CAD build for the part. Positions are in the model's coordinates, mm. Face numbers are marked on the shaded views. A direction names the side the tool comes from. Round coordinates to 2 decimals unless told otherwise and drop trailing zeros. Order: outer loops, then holes, each group sorted by start corner. A loop starts at its lowest first (then second) coordinate and runs counter-clockwise, first axis right, second up. Notation, with made-up numbers: M 23,10.25 L 62,10.25 A16 ccw 62,39.25 Z; hole C -16,5 d9. An arc over 180 degrees is marked long. Put each result on its own line as item: value.
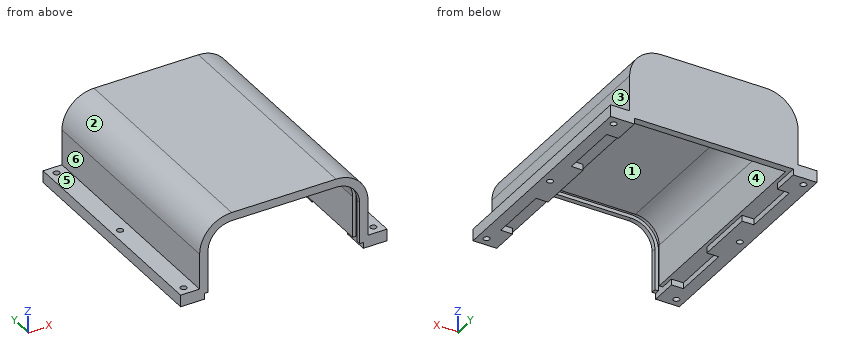
```python
from build123d import *

# Parameters (mm, degrees)
SKETCH_W        = 174
SKETCH_H        = 195
SKETCH_R        = 2.6
PAD_DEPTH       = 10
PAD001_DEPTH    = 195
POCKET_DEPTH    = 5
POCKET_FACE10_W = 195
POCKET_FACE10_H = 128
POCKET001_DEPTH = 5
PAD003_DEPTH    = 6
POCKET003_DEPTH = 10
PAD006_DEPTH    = 4


with BuildPart() as part:
    # Sketch → Pad (new body)
    with BuildSketch(Plane.XY):
        Rectangle(SKETCH_W, SKETCH_H)
        with Locations((80, 90)):
            Circle(SKETCH_R, mode=Mode.SUBTRACT)
        with Locations((-80, 90)):
            Circle(SKETCH_R, mode=Mode.SUBTRACT)
        with Locations((-80, -90)):
            Circle(SKETCH_R, mode=Mode.SUBTRACT)
        with Locations((80, -90)):
            Circle(SKETCH_R, mode=Mode.SUBTRACT)
        with Locations((-80, 0)):
            Circle(SKETCH_R, mode=Mode.SUBTRACT)
        with Locations((80, 0)):
            Circle(SKETCH_R, mode=Mode.SUBTRACT)
    extrude(amount=PAD_DEPTH)

    # Sketch001 (on Face3 of Pad) → Pad001 (join)
    with BuildSketch(Plane.XZ.offset(97.5)):
        with BuildLine():
            Line((-64, 10), (-64, 40))
            ThreePointArc((-44, 60), (-58.142136, 54.142136), (-64, 40))
            Line((-44, 60), (44, 60))
            ThreePointArc((64, 40), (58.142136, 54.142136), (44, 60))
            Line((64, 40), (64, 10))
            Line((64, 10), (71, 10))
            Line((71, 40), (71, 10))
            ThreePointArc((71, 40), (63.091883, 59.091883), (44, 67))
            Line((-44, 67), (44, 67))
            ThreePointArc((-44, 67), (-63.091883, 59.091883), (-71, 40))
            Line((-71, 10), (-71, 40))
            Line((-64, 10), (-71, 10))
        make_face()
    extrude(amount=-PAD001_DEPTH)

    # Sketch003 (on Face4 of Pad001) → Pocket (cut)
    with BuildSketch(Plane(origin=(0, 0, 0), x_dir=(1, 0, 0), z_dir=(0, 0, -1))):
        Polygon((-67, 97.5), (67, 97.5), (67, 75), (77, 75), (77, 25), (67, 25), (67, 0), (67, -25), (77, -25), (77, -75), (67, -75), (67, -97.5), (-67, -97.5), (-67, -75), (-77, -75), (-77, -25), (-67, -25), (-67, 0), (-67, 25), (-77, 25), (-77, 75), (-67, 75), align=None)
    extrude(amount=-POCKET_DEPTH, mode=Mode.SUBTRACT)

    # Pocket Face10 → Pocket001 (cut)
    with BuildSketch(Plane(origin=(0, 0, 10), x_dir=(0, 1, 0), z_dir=(0, 0, 1))):
        Rectangle(POCKET_FACE10_W, POCKET_FACE10_H)
    extrude(amount=-POCKET001_DEPTH, mode=Mode.SUBTRACT)

    # Sketch005 (on Face6 of Pocket001) → Pad003 (join)
    with BuildSketch(Plane(origin=(0, 97.5, 0), x_dir=(-1, 0, 0), z_dir=(0, 1, 0))):
        with BuildLine():
            Line((-64, 5), (64, 5))
            Line((64, 40), (64, 5))
            ThreePointArc((64, 40), (58.142143, 54.142129), (44.00002, 60))
            Line((-44, 60), (44.00002, 60))
            ThreePointArc((-44, 60), (-58.142136, 54.142136), (-64, 40))
            Line((-64, 40), (-64, 5))
        make_face()
    extrude(amount=-PAD003_DEPTH)

    # Sketch006 (on Face30 of Pad003) → Pocket003 (cut)
    with BuildSketch(Plane.XZ.offset(97.5)):
        with BuildLine():
            ThreePointArc((-44, 63), (-60.263456, 56.263456), (-67, 40))
            Line((-67, 40), (-67, 0))
            Line((-67, 0), (67, 0))
            Line((67, 0), (67, 40))
            ThreePointArc((67, 40), (60.263456, 56.263456), (44, 63))
            Line((-44, 63), (44, 63))
        make_face()
    extrude(amount=-POCKET003_DEPTH, mode=Mode.SUBTRACT)

    # Sketch008 (on Face33 of Pocket003) → Pad006 (join)
    with BuildSketch(Plane.XZ.offset(97.5)):
        with BuildLine():
            Line((-44, 63), (44, 63))
            ThreePointArc((67, 40), (60.263456, 56.263456), (44, 63))
            Line((67, 5), (67, 40))
            Line((64, 5), (67, 5))
            Line((64, 5), (64, 40))
            ThreePointArc((64, 40), (58.142136, 54.142136), (44, 60))
            Line((44, 60), (-44, 60))
            ThreePointArc((-44, 60), (-58.142136, 54.142136), (-64, 40))
            Line((-64, 40), (-64, 5))
            Line((-64, 5), (-67, 5))
            Line((-67, 40), (-67, 5))
            ThreePointArc((-44, 63), (-60.263456, 56.263456), (-67, 40))
        make_face()
    extrude(amount=-PAD006_DEPTH)


solid = part.part
```
Item 1: Band-saw the part on D-D on z = 26.5. Give the cut face in (x, y).
Answers below:
outline: M -71,-97.5 L -64,-97.5 L -64,-93.5 L -67,-93.5 L -67,-87.5 L -64,-87.5 L -64,91.5 L 64,91.5 L 64,-87.5 L 67,-87.5 L 67,-93.5 L 64,-93.5 L 64,-97.5 L 71,-97.5 L 71,97.5 L -71,97.5 Z
Item 2: Band-saw the part on B-B on x = 80. Give the cut face in (y, z), and give its area (3 significant figures).
Answers below:
outline: M -97.5,0 L -92.6,0 L -92.6,10 L -97.5,10 Z; M -87.4,0 L -2.6,0 L -2.6,10 L -87.4,10 Z; M 2.6,0 L 87.4,0 L 87.4,10 L 2.6,10 Z; M 92.6,0 L 97.5,0 L 97.5,10 L 92.6,10 Z
area: 1,790 mm²
Item 3: Probe line 1 along Y through (x, z) = (-80, 8); line 2 along X through (y, z) = (41.5, 19); line 3 along Z through (x, y) = (-22.5, 11). List the from-to ranges inside material, lowest first. Write a range as [from, to].
Answers below:
line 1: [-97.5, -92.6], [-87.4, -2.6], [2.6, 87.4], [92.6, 97.5]
line 2: [-71, -64], [64, 71]
line 3: [60, 67]
Item 4: Pin check, flat tips, straight feed: P1, Ø8, axis at x = 45.5, z = 51, coming from the -Y side; P2, Ø2.5, axis at x = 66, y = -95.5, coming from the -Z side; P3, Ø24, axis at y = -7.5, z = 29, coming from the +X side; P4, Ø5, axis at x = -6, y = -90.5, coming from the -Z side. Stop position of each tip, or through.
Answers below:
P1: y = 91.5
P2: z = 0
P3: x = 71
P4: z = 63
Item 5: Band-saw the part on A-A on y = 0. Give the cut face in (x, z).
Answers below:
outline: M -87,0 L -82.6,0 L -82.6,10 L -87,10 Z; M -77.4,0 L -67,0 L -67,5 L -64,5 L -64,40 A20 cw -44,60 L 44,60 A20 cw 64,40 L 64,5 L 67,5 L 67,0 L 77.4,0 L 77.4,10 L 71,10 L 71,40 A27 ccw 44,67 L -44,67 A27 ccw -71,40 L -71,10 L -77.4,10 Z; M 82.6,0 L 87,0 L 87,10 L 82.6,10 Z
Item 6: Tool access for the marked faces 1, 2 and 3: list every direction of +Z, -Z, +X, -X, +Y, -Y with a clear straight run to the whole face (end or side of a thin tool).
Answers below:
face 1: -Z, -Y
face 2: +Z, -X, +Y, -Y
face 3: +Z, +X, +Y, -Y
Item 7: Band-saw the part on C-C on x = 19. Give the cut face in (y, z), and give its area (3 significant figures).
Answers below:
outline: M -97.5,60 L -93.5,60 L -93.5,63 L -87.5,63 L -87.5,60 L 91.5,60 L 91.5,5 L 97.5,5 L 97.5,67 L -97.5,67 Z
area: 1,680 mm²
Item 8: Mould opens along X. For the marked faces 4, 5 and 6 say: pulls with the +X half, pulls with the -X half, needs draft (parallel to the pull), parting line crosses it, or undercut.
Answers below:
face 4: undercut
face 5: needs draft
face 6: pulls with the -X half
